Autodesk Inventor part; units mm, degrees
ref_plane "YZ Plane" through (0, 0, 0) normal (1, 0, 0) x (0, 1, 0)
ref_plane "XZ Plane" through (0, 0, 0) normal (0, 1, 0) x (-1, 0, 0)
ref_plane "XY Plane" through (0, 0, 0) normal (0, 0, 1) x (1, 0, 0)
sketch "Sketch1" plane through (0, 0, 0) normal (0, 0, 1) x (1, 0, 0)
  line L0 (0, 6.35) -> (0, 53.34)
  line L1 (0, 53.34) -> (-19.05, 53.34)
  line L2 (-19.05, 53.34) -> (-19.05, 55.245)
  line L3 (-12.7, 48.895) -> (-6.35, 48.895)
  line L4 (-6.35, 48.895) -> (-6.35, 13.335)
  line L5 (-6.35, 13.335) -> (-19.05, 13.335)
  line L6 (-19.05, 13.335) -> (-19.05, 12.7)
  line L7 (-12.7, 8.89) -> (-6.35, 8.89)
  line L8 (-6.35, 8.89) -> (-6.35, 0)
  line L9 (-6.35, 0) -> (0, 0)
  line L10 (-19.05, 55.245) -> (-19.05, 40.005)
  line L11 (-19.05, 40.005) -> (-12.7, 40.005)
  line L12 (-12.7, 40.005) -> (-12.7, 48.895)
  line L13 (-19.05, 12.7) -> (-19.05, 0)
  line L14 (-19.05, 0) -> (-12.7, 0)
  line L15 (-12.7, 0) -> (-12.7, 8.89)
  line L16 (0, 0) -> (38.1, 0)
  line L17 (38.1, 0) -> (38.1, 6.35)
  line L18 (38.1, 6.35) -> (0, 6.35)
  point P0 (-19.05, 53.34)
  point P1 (-19.05, 11.43)
  dimension "d1" = 35.56
  dimension "d2" = 4.445
  dimension "d3" = 4.445
  dimension "d4" = 6.35
  dimension "d6" = 6.35
  dimension "d7" = 6.35
  dimension "d10" = 38.1
  dimension "d13" = 13.335
  dimension "d14" = 13.335
extrude "Extrusion1" add sketch "Sketch1" along normal mid plane 3.81
equation "\"d11\" = width"
equation "\"width\" = 3.81"
properties part number "basicHangerV01"
Could you check a few things on this model? Use its own coordinates, in mm. A direction names the side the tool comes from. Coordinates: 2 decimals unless noted, no trailing zeros. Write each loop counter-clockwise with the first axis right and the second up, starting at its lowest first coordinate (ties: lowest second). Pieces come first, ordered by that corner, then holes. Notation, with made-up numbers: (8.25, -24) -> (13.25, -24) arc R19 ccw to (13.25, 7) -> close; hole circle Ø5 at (2, -21.75). An arc over 180 degrees is marked (long way). Write item = value, one per line. Start each with the question number.
(1) I want a section at B-B (y = 3.5). Please give me the cut outline in (x, z) (3 decimals).
(2) I want a section at C-C (z = 0.05). Please give me the cut outline in (x, y) (3 decimals), plus the area to 3 significant figures.
(3) I want a section at A-A (x = -14). Please give me the cut outline in (y, z) (3 decimals).
(4) I need wall thicknesses on line 1 (X direction, y = 43, z = 0.3); line 2 (Y direction, x = 10.5, z = -0.15); line 3 (Y direction, x = -8.5, z = -1) (3 decimals). Which ranges of each line are inside material? Lowest first, please. Write a range as [from, to].
(5) Will these pins go through, and if not, where does the flat tip stop? pin 1 (1.5 mm diameter, centred on y = 32.5, z = -1, fed in from -X); pin 2 (1.9 mm diameter, centred on y = 36.5, z = 1, fed in from +X).
(6) I want a section at D-D (y = 33.5). Please give me the cut outline in (x, z) (3 decimals).
(7) Which directions (+Z, -Z, +X, -X, +Y, -Y) give clear straight access to the entire face, cutting with the end or side of a thin tool? Please do faces 4 (the face through (-16, 40.005, 0)), 5 (the face through (0, 30, 0)), 6 (the face through (-12.7, 44, 0)), 7 (the face through (-12.7, 4, 0)).
(8) We'd pull the mould along X, two halves only. Please class faces 1 (the face through (19, 6.35, 0)), 2 (the face through (-10, 8.89, 0)), 3 (the face through (-19.05, 7, 0)): released by +X, released by -X, zero draft, split by the parting line, or undercut.
Result set:
q1.outline = (-19.05, -1.905) -> (-12.7, -1.905) -> (-12.7, 1.905) -> (-19.05, 1.905) -> close; (-6.35, -1.905) -> (38.1, -1.905) -> (38.1, 1.905) -> (-6.35, 1.905) -> close
q2.outline = (-19.05, 0) -> (-12.7, 0) -> (-12.7, 8.89) -> (-6.35, 8.89) -> (-6.35, 0) -> (38.1, 0) -> (38.1, 6.35) -> (0, 6.35) -> (0, 53.34) -> (-19.05, 53.34) -> (-19.05, 40.005) -> (-12.7, 40.005) -> (-12.7, 48.895) -> (-6.35, 48.895) -> (-6.35, 13.335) -> (-19.05, 13.335) -> close
q2.area = 806 mm2
q3.outline = (0, -1.905) -> (13.335, -1.905) -> (13.335, 1.905) -> (0, 1.905) -> close; (40.005, -1.905) -> (53.34, -1.905) -> (53.34, 1.905) -> (40.005, 1.905) -> close
q4.line_1 = [-19.05, -12.7], [-6.35, 0]
q4.line_2 = [0, 6.35]
q4.line_3 = [8.89, 13.335], [48.895, 53.34]
q5.pin_1 = -6.35
q5.pin_2 = 0
q6.outline = (-6.35, -1.905) -> (0, -1.905) -> (0, 1.905) -> (-6.35, 1.905) -> close
q7.face_4 = +Z, -Z, -X
q7.face_5 = +Z, -Z, +X, +Y
q7.face_6 = +Z, -Z
q7.face_7 = +Z, -Z, -Y
q8.face_1 = zero draft
q8.face_2 = undercut
q8.face_3 = released by -X
